CAD build for the part. Positions are in the model's coordinates, mm. Round coordinates to 2 decimals unless told otherwise and drop trailing zeros. Write each loop counter-clockwise with the first axis right and the second up, starting at its lowest first coordinate (ties: lowest second). Pieces come first, ordered by that corner, then holes. Notation, with made-up numbers: (-39, 47.25) -> (-18, 47.25) arc R18 ccw to (-18, 57.25) -> close; hole circle Ø8 at (0.25, 63). An arc over 180 degrees is marked (long way). Answer in a Markdown table with one row per item. Add a question column.
```python
from build123d import *

# Parameters (mm, degrees)
BOSS_EXTRUDE1_DEPTH       = 6
SKETCH4_R                 = 0.495653738
CUT_EXTRUDE3_DEPTH        = 10
BOSS_EXTRUDE3_DEPTH       = 6
SKETCH6_R                 = 2
SKETCH6_R_2               = 4
CUT_EXTRUDE4_DEPTH        = 12
CIRPATTERN1_COUNT         = 4
BOSS_EXTRUDE4_DEPTH       = 6
F_4_0MM_DOWEL_HOLE4_D     = 4
F_4_0MM_DOWEL_HOLE4_DEPTH = 98.31
F_4_0MM_DOWEL_HOLE4_TIP   = 1.201721238
F_4_0MM_DOWEL_HOLE5_D     = 4
F_4_0MM_DOWEL_HOLE5_DEPTH = 98.31
F_4_0MM_DOWEL_HOLE5_TIP   = 1.201721238
SKETCH34_W                = 35.409448417
SKETCH34_H                = 30.185103568
SKETCH34_W_2              = 36.570413939
SKETCH34_H_2              = 111.452690099
SKETCH34_W_3              = 29.604620807
SKETCH34_H_3              = 33.087517373
SKETCH34_W_4              = 33.087517373
SKETCH34_W_5              = 27.282689764
SKETCH34_H_4              = 24.96075872
SKETCH34_W_6              = 20.316896633
SKETCH34_H_5              = 92.296758988
SKETCH34_W_7              = 27.863172524
SKETCH34_H_6              = 11.609655218
SKETCH34_W_8              = 24.025079094
SKETCH34_H_7              = 13.26196209
SKETCH34_W_9              = 25.256962543
SKETCH34_H_8              = 14.571324544
SKETCH34_W_10             = 26.74183209
SKETCH34_H_9              = 13.599902908
SKETCH34_W_11             = 6.832653797
SKETCH34_H_10             = 26.571431431
SKETCH34_W_12             = 13.665307593
SKETCH34_H_11             = 29.608166452
SKETCH34_W_13             = 111.542887187
SKETCH34_H_12             = 48.356959239
SKETCH34_W_14             = 14.599955316
SKETCH34_H_13             = 35.285066425
SKETCH34_W_15             = 19.210467522
SKETCH34_H_14             = 26.471341651
SKETCH34_W_16             = 101.584483163
SKETCH34_H_15             = 31.891508091
SKETCH34_W_17             = 12.108434582
SKETCH34_H_16             = 29.018914361
SKETCH34_W_18             = 8.981277634
SKETCH34_H_17             = 24.21737362
SKETCH34_W_19             = 29.087219519
SKETCH34_H_18             = 16.362951604
SKETCH34_W_20             = 17.661842556
SKETCH34_H_19             = 22.206862892
SKETCH34_W_21             = 25.871946372
SKETCH34_W_22             = 23.792293824
SKETCH34_H_20             = 9.539966182
SKETCH34_H_21             = 15.633594749
SKETCH34_W_23             = 12.316273022
SKETCH34_H_22             = 19.237958234
BOSS_EXTRUDE5_DEPTH       = 6


with BuildPart() as part:
    # Sketch1 → Boss-Extrude1 (new body)
    with BuildSketch(Plane(origin=(0, 0, 0), x_dir=(1, 0, 0), z_dir=(0, 1, 0))):
        with BuildLine():
            Line((-110, 50), (-300, 50))
            ThreePointArc((-300, 50), (-307.071067812, 47.071067812), (-310, 40))
            Line((-310, 40), (-310, -40))
            ThreePointArc((-310, -40), (-307.071067812, -47.071067812), (-300, -50))
            Line((-300, -50), (-110, -50))
            Line((-110, -50), (-60, -100))
            Line((-60, -100), (-60, -290))
            ThreePointArc((-60, -290), (-57.071067812, -297.071067812), (-50, -300))
            Line((-50, -300), (30, -300))
            ThreePointArc((30, -300), (37.071067812, -297.071067812), (40, -290))
            Line((40, -290), (40, -100))
            Line((40, -100), (90, -50))
            Line((90, -50), (280, -50))
            ThreePointArc((280, -50), (287.071067812, -47.071067812), (290, -40))
            Line((290, -40), (290, 40))
            ThreePointArc((290, 40), (287.071067812, 47.071067812), (280, 50))
            Line((280, 50), (90, 50))
            Line((90, 50), (40, 100))
            Line((40, 100), (40, 290))
            ThreePointArc((40, 290), (37.071067812, 297.071067812), (30, 300))
            Line((30, 300), (-50, 300))
            ThreePointArc((-50, 300), (-57.071067812, 297.071067812), (-60, 290))
            Line((-60, 290), (-60, 100))
            Line((-60, 100), (-110, 50))
        make_face()
    extrude(amount=BOSS_EXTRUDE1_DEPTH)

    # Sketch4 → Cut-Extrude3 (cut)
    with BuildSketch(Plane(origin=(0, 6, 0), x_dir=(1, 0, 0), z_dir=(0, 1, 0))):
        with Locations(Location((-10, 0, 0), (0, 0, 270))):
            Circle(SKETCH4_R)
    extrude(amount=-CUT_EXTRUDE3_DEPTH, mode=Mode.SUBTRACT)

    # Sketch5 → Boss-Extrude3 (add)
    with BuildSketch(Plane(origin=(0, 6, 0), x_dir=(1, 0, 0), z_dir=(0, 1, 0))):
        Polygon((-300, 50), (-60, 290), (-60, 240), (-250, 50), align=None)
        Polygon((40, 290), (280, 50), (230, 50), (40, 240), align=None)
        Polygon((280, -50), (40, -290), (40, -240), (230, -49.07797178), align=None)
        Polygon((-300, -50), (-60, -290), (-60, -240), (-250, -50), align=None)
    extrude(amount=-BOSS_EXTRUDE3_DEPTH)

    # Sketch6 → Cut-Extrude4 (cut)
    with BuildSketch(Plane(origin=(0, 6, 0), x_dir=(1, 0, 0), z_dir=(0, 1, 0))):
        with Locations(Location((-37.824146891, 287.83697558, 0), (0, 0, 270))):
            Circle(SKETCH6_R)
        with Locations(Location((-37.824146891, 272.83697558, 0), (0, 0, 270))):
            Circle(SKETCH6_R)
        with Locations(Location((-46.483109463, 221.536893944, 0), (0, 0, 270))):
            Circle(SKETCH6_R)
        with Locations(Location((-46.483109463, 135.06793836, 0), (0, 0, 270))):
            Circle(SKETCH6_R)
        with Locations(Location((-69.817594081, 73.334484618, 0), (0, 0, 270))):
            Circle(SKETCH6_R)
        with Locations(Location((49.817594081, 73.334484618, 0), (0, 0, 270))):
            Circle(SKETCH6_R)
        with Locations(Location((26.483109463, 135.06793836, 0), (0, 0, 270))):
            Circle(SKETCH6_R)
        with Locations(Location((26.483109463, 221.536893944, 0), (0, 0, 270))):
            Circle(SKETCH6_R)
        with Locations(Location((191.360389693, 113.639610307, 0), (0, 0, 270))):
            Circle(SKETCH6_R)
        with Locations(Location((128.639610307, 176.360389693, 0), (0, 0, 270))):
            Circle(SKETCH6_R)
        with Locations(Location((17.824146891, 272.83697558, 0), (0, 0, 270))):
            Circle(SKETCH6_R)
        with Locations(Location((17.824146891, 287.83697558, 0), (0, 0, 270))):
            Circle(SKETCH6_R)
        with Locations(Location((-10, 0, 0), (0, 0, 270))):
            Circle(SKETCH6_R_2)
    cut_extrude4 = extrude(amount=-CUT_EXTRUDE4_DEPTH, mode=Mode.SUBTRACT)

    # CirPattern1: Cut-Extrude4 ×4 about axis
    cirpattern1_axis = Axis((-10, 0, 0), (0, 1, 0))
    for i in range(1, CIRPATTERN1_COUNT):
        add(cut_extrude4.rotate(cirpattern1_axis, i * 360 / CIRPATTERN1_COUNT), mode=Mode.SUBTRACT)

    # Sketch7 → Boss-Extrude4 (add)
    with BuildSketch(Plane(origin=(0, 6, 0), x_dir=(1, 0, 0), z_dir=(0, 1, 0))):
        Polygon((40, 240), (230, 50), (90, 50), (40, 100), align=None)
        Polygon((90, -50), (229.082424571, -50), (40, -240), (40, -100), align=None)
        Polygon((-60, 240), (-60, 100), (-110, 50), (-250, 50), align=None)
        Polygon((-110, -50), (-60, -100), (-60, -240), (-250, -50), align=None)
    extrude(amount=-BOSS_EXTRUDE4_DEPTH)

    # Ø4.0mm Dowel Hole4
    with Locations(Plane(origin=(0, 0, 0), x_dir=(-1, 0, 0), z_dir=(0, -1, 0))):
        with Locations((46.483109463, -278), (-26.483109463, -278), (-268, -36.483109463), (-268, 36.483109463), (-26.483109463, 278), (46.483109463, 278), (288, 36.483109463), (288, -36.483109463)):
            Hole(F_4_0MM_DOWEL_HOLE4_D / 2, depth=F_4_0MM_DOWEL_HOLE4_DEPTH)
            with Locations((0, 0, -(F_4_0MM_DOWEL_HOLE4_DEPTH + F_4_0MM_DOWEL_HOLE4_TIP / 2))):  # 118° drill point
                Cone(0, F_4_0MM_DOWEL_HOLE4_D / 2, F_4_0MM_DOWEL_HOLE4_TIP, mode=Mode.SUBTRACT)

    # Ø4.0mm Dowel Hole5
    with Locations(Plane(origin=(0, 6, 0), x_dir=(1, 0, 0), z_dir=(0, 1, 0))):
        with Locations((-30.430566073, -32.5), (31.383083735, -32.5), (31.383083735, 32.5), (-30.430566073, 32.5)):
            Hole(F_4_0MM_DOWEL_HOLE5_D / 2, depth=F_4_0MM_DOWEL_HOLE5_DEPTH)
            with Locations((0, 0, -(F_4_0MM_DOWEL_HOLE5_DEPTH + F_4_0MM_DOWEL_HOLE5_TIP / 2))):  # 118° drill point
                Cone(0, F_4_0MM_DOWEL_HOLE5_D / 2, F_4_0MM_DOWEL_HOLE5_TIP, mode=Mode.SUBTRACT)

    # Sketch34 → Boss-Extrude5 (add)
    with BuildSketch(Plane(origin=(0, 6, 0), x_dir=(1, 0, 0), z_dir=(0, 1, 0))):
        with Locations((-78.80313436, 68.745934319)):
            Rectangle(SKETCH34_W, SKETCH34_H)
        with Locations((-144.397686345, -2.072962514)):
            Rectangle(SKETCH34_W_2, SKETCH34_H_2)
        with Locations((-75.900720554, -65.635824837)):
            Rectangle(SKETCH34_W_3, SKETCH34_H_3)
        with Locations((57.029831699, -65.635824837)):
            Rectangle(SKETCH34_W_4, SKETCH34_H_3)
        with Locations((59.932245503, 66.133761895)):
            Rectangle(SKETCH34_W_5, SKETCH34_H_4)
        with Locations((127.268245772, 1.700175431)):
            Rectangle(SKETCH34_W_6, SKETCH34_H_5)
        with Locations((-288.647652436, 25.79021001)):
            Rectangle(SKETCH34_W_7, SKETCH34_H_6)
        with Locations((-290.566699151, -25.743228086)):
            Rectangle(SKETCH34_W_8, SKETCH34_H_7)
        with Locations((-207.82626231, -113.697936261)):
            Rectangle(SKETCH34_W_9, SKETCH34_H_8)
        with Locations((-149.311977269, -174.411788529)):
            Rectangle(SKETCH34_W_10, SKETCH34_H_9)
        with Locations((-37.704576229, -280.142299522)):
            Rectangle(SKETCH34_W_11, SKETCH34_H_10)
        with Locations((16.577062267, -278.623932011)):
            Rectangle(SKETCH34_W_12, SKETCH34_H_11)
        with Locations((-15.285370581, -137.876415881)):
            Rectangle(SKETCH34_W_13, SKETCH34_H_12)
        with Locations((102.99002157, -192.054321742)):
            Rectangle(SKETCH34_W_14, SKETCH34_H_13)
        with Locations((162.158261537, -134.219269359)):
            Rectangle(SKETCH34_W_15, SKETCH34_H_14)
        with Locations((-10.306168569, 138.617659885)):
            Rectangle(SKETCH34_W_16, SKETCH34_H_15)
        with Locations((-35.066685836, 277.003869093)):
            Rectangle(SKETCH34_W_17, SKETCH34_H_16)
        with Locations((17.598670848, 280.473392986)):
            Rectangle(SKETCH34_W_18, SKETCH34_H_17)
        with Locations((-180.654171279, 134.499996933)):
            Rectangle(SKETCH34_W_19, SKETCH34_H_18)
        with Locations((-117.281558097, 197.029847706)):
            Rectangle(SKETCH34_W_20, SKETCH34_H_19)
        with Locations((271.071548242, 25.79021001)):
            Rectangle(SKETCH34_W_21, SKETCH34_H_6)
        with Locations((270.031721968, -27.60422604)):
            Rectangle(SKETCH34_W_22, SKETCH34_H_20)
        with Locations((127.268245772, 172.147264617)):
            Rectangle(SKETCH34_W_6, SKETCH34_H_21)
        with Locations((187.981166364, 113.052926722)):
            Rectangle(SKETCH34_W_23, SKETCH34_H_22)
    extrude(amount=-BOSS_EXTRUDE5_DEPTH)


solid = part.part
```
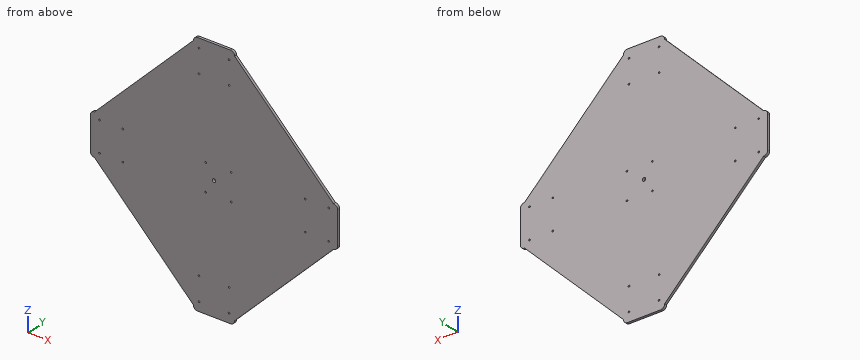
Item 1: Drill centre lines: probe 1 along X at (y, z) = (2.85, -32.5); probe 2 along Z at (x, y) = (-288, 2.7); probe 3 along X at (y, z) = (4.2, 0). Where is each one in solid material? Low to high.
Item 2: Saw through at B-B on z = -197.5. Give the cut face in (x, y).
Item 3: Saw through at C-C on y = 2.6. Count the separate pieces of the cut face and the enclosed holes in it, then the cut area to 3 significant figures.
Item 4: Saw through at A-A on x = 164.5. Give the cut face in (y, z), then the cut area to 3 significant figures.
Item 5: Pin check, flat tips, straight feed: pin 1 (5 mm diameter, centred on x = -46.48, z = 278, fed in from -Y); pin 2 (3.5 mm diameter, centred on x = 268, z = -36.48, fed in from +Y). Stop position of each tip, or through.
Recorded:
| question | item | result |
|---|---|---|
| 1 | probe 1 | -310 to -32.43, -28.43 to 29.38, 33.38 to 290 |
| 1 | probe 2 | -62 to -38.48, -34.48 to 34.48, 38.48 to 62 |
| 1 | probe 3 | -310 to -14, -6 to 290 |
| 2 | outline | (-152.5, 0) -> (132.5, 0) -> (132.5, 6) -> (-152.5, 6) -> close |
| 3 | separate pieces | 1 |
| 3 | enclosed holes | 21 |
| 3 | area | 225,000 mm2 |
| 4 | outline | (0, -165.5) -> (6, -165.5) -> (6, 165.5) -> (0, 165.5) -> close |
| 4 | area | 1,990 mm2 |
| 5 | pin 1 | y = 0 |
| 5 | pin 2 | through |
